Work out the finished part from the listing and answer in its coordinate system (mm). A direction names the side the tool comes from. Give positions to 0.01 mm unless a question says otherwise; leave off trailing zeros. Loops run counter-clockwise (first coordinate to the right, second up) from the corner with the lowest first, then second, coordinate; pieces in that order, holes last.
Autodesk Inventor part; units mm, degrees
ref_plane "YZ Plane" through (0, 0, 0) normal (1, 0, 0) x (0, 1, 0)
ref_plane "XZ Plane" through (0, 0, 0) normal (0, 1, 0) x (-1, 0, 0)
ref_plane "XY Plane" through (0, 0, 0) normal (0, 0, 1) x (1, 0, 0)
sketch "Sketch1" plane through (0, 0, 0) normal (0, 1, 0) x (-1, 0, 0)
  circle A0 centre (0, 0) radius 35
  line L0 (0, 0) -> (0, -22)
  circle A1 centre (0, -22) radius 8.5
  circle A2 centre (-19.0526, -11) radius 8.5
  circle A3 centre (-19.0526, 11) radius 8.5
  circle A4 centre (0, 22) radius 8.5
  circle A5 centre (19.0526, 11) radius 8.5
  circle A6 centre (19.0526, -11) radius 8.5
  line L1 (-2.39, 0.895) -> (2.39, 0.895)
  line L2 (2.39, 0.895) -> (2.39, -0.895)
  line L3 (2.39, -0.895) -> (-2.39, -0.895)
  line L4 (-2.39, -0.895) -> (-2.39, 0.895)
  line L5 (-2.39, 0.895) -> (2.39, -0.895) construction
  line L6 (2.39, 0.895) -> (-2.39, -0.895) construction
  line L7 (-0.895, -2.39) -> (-0.895, 2.39)
  line L8 (0.895, -2.39) -> (-0.895, -2.39)
  line L9 (-0.895, 2.39) -> (0.895, 2.39)
  line L10 (0.895, 2.39) -> (0.895, -2.39)
  line L11 (-0.895, -2.39) -> (0.895, 2.39) construction
  line L12 (-0.895, 2.39) -> (0.895, -2.39) construction
  line L13 (2.39, -0.895) -> (-2.39, -0.895)
  line L14 (2.39, 0.895) -> (2.39, -0.895)
  line L15 (-2.39, -0.895) -> (-2.39, 0.895)
  line L16 (-2.39, 0.895) -> (2.39, 0.895)
  line L17 (2.39, -0.895) -> (-2.39, 0.895) construction
  line L18 (-2.39, -0.895) -> (2.39, 0.895) construction
  line L19 (0.895, 2.39) -> (0.895, -2.39)
  line L20 (-0.895, 2.39) -> (0.895, 2.39)
  line L21 (0.895, -2.39) -> (-0.895, -2.39)
  line L22 (-0.895, -2.39) -> (-0.895, 2.39)
  line L23 (0.895, 2.39) -> (-0.895, -2.39) construction
  line L24 (0.895, -2.39) -> (-0.895, 2.39) construction
  point P0 (-0.895, -0.895)
  point P1 (-0.895, 0.895)
  point P2 (0.895, 0.895)
  point P3 (0.895, -0.895)
  dimension "d0" = 70
  dimension "d1" = 22
  dimension "d2" = 17
  dimension "d5" = 360
  dimension "d9" = 4.78
  dimension "d10" = 1.79
  dimension "d13" = 360
extrude "Extrusion1" add sketch "Sketch1" along normal blind 4
properties part number "disc_mover"
Item 1: For faces 4 (the face through (0, 4, -7)), 5 (the face through (-2.39, 2, 0)), determine the directions among +Z, -Z, +X, -X, +Y, -Y from which every point of the face is accessible in a straight line to the end or side of a thin tool.
Item 2: Find section B-B, the plane x = 0. Write down the section's boundary in (y, z), plus the area to 3 significant figures.
Item 3: Consider line 1 (Z direction, x = 0, y = 2.35); line 2 (Z direction, x = 22, y = 2.15); line 3 (Z direction, x = -12, y = 0.8). Determine where each line is inside the solid, lowest interval first.
Item 4: Flat-ended cylindrical pins translate along their axes: pin 1 Ø0.5 at (x, y) = (0, 1.5) entering from +Z; pin 2 Ø0.7 at (y, z) = (2, -1.5) entering from +X; pin 3 Ø0.7 at (y, z) = (1.5, -1.5) entering from -X. Find the tip coordinate at first contact, or state that the pin passes through.
Item 5: Find section C-C, the plane y = 0.9. Write down the section's boundary in (x, z) (3 decimals).
Item 6: Find section A-A, the plane z = 0. Write down the section's boundary in (x, y), plus the area to 3 significant figures.
Item 7: Determine the mould class of faces 1 (the face through (28, 2, 21)), 2 (the face through (-2, 2, -0.895)), 3 (the face through (0, 0, -7)) for opening direction Z: released by +Z, released by -Z, zero draft, split by the parting line, or undercut.
Item 8: Find section D-D, the plane x = -23. Write down the section's boundary in (y, z), plus the area to 3 significant figures.
Ans:
1. face 4: +Z, -Z, +X, -X, +Y
1. face 5: +Y, -Y
2. outline: (0, -35) - (4, -35) - (4, -30.5) - (0, -30.5) - close; (0, -13.5) - (4, -13.5) - (4, -2.39) - (0, -2.39) - close; (0, 2.39) - (4, 2.39) - (4, 13.5) - (0, 13.5) - close; (0, 30.5) - (4, 30.5) - (4, 35) - (0, 35) - close
2. area: 125 mm2
3. line 1: z = -35 to -30.5, -13.5 to -2.39, 2.39 to 13.5, 30.5 to 35
3. line 2: z = -27.22 to -18.97, -3.03 to 3.03, 18.97 to 27.22
3. line 3: z = -32.88 to -15.74, -6.26 to 6.26, 15.74 to 32.88
4. pin 1: stops at z = 35
4. pin 2: stops at x = 34.98
4. pin 3: stops at x = -34.98
5. outline: circle Ø70 at (0, 0); hole circle Ø17 at (-19.053, -11); hole circle Ø17 at (-19.053, 11); hole circle Ø17 at (0, -22); hole circle Ø17 at (0, 22); hole (-2.39, -0.895) - (-0.895, -0.895) - (-0.895, -2.39) - (0.895, -2.39) - (0.895, -0.895) - (2.39, -0.895) - (2.39, 0.895) - (0.895, 0.895) - (0.895, 2.39) - (-0.895, 2.39) - (-0.895, 0.895) - (-2.39, 0.895) - close; hole circle Ø17 at (19.053, -11); hole circle Ø17 at (19.053, 11)
6. outline: (-35, 0) - (-2.39, 0) - (-2.39, 4) - (-35, 4) - close; (2.39, 0) - (35, 0) - (35, 4) - (2.39, 4) - close
6. area: 261 mm2
7. face 1: split by the parting line
7. face 2: undercut
7. face 3: zero draft
8. outline: (0, -26.38) - (4, -26.38) - (4, -18.53) - (0, -18.53) - close; (0, -3.47) - (4, -3.47) - (4, 3.47) - (0, 3.47) - close; (0, 18.53) - (4, 18.53) - (4, 26.38) - (0, 26.38) - close
8. area: 90.6 mm2
